Read the model definition and answer for the solid it produces. Units are mm, in the model's axes. A direction names the side the tool comes from. Coordinates: 2 decimals unless noted, no trailing zeros. Write each loop counter-clockwise with the first axis right and the second up, starting at its lowest first coordinate (ties: lowest second). Pieces come first, ordered by that corner, then holes.
Item 1: Each of these flat-tipped pins is pushed along its axis until it touches: P1, Ø10, axis at x = 77, z = -24, coming from the +Y side; P2, Ø1.5, axis at y = 14, z = -18.5, coming from the -X side; P3, Ø21, axis at x = 97, z = -25, coming from the -Y side. Where does it stop, or does it pass through?
Item 2: Straight lines are drawn through the part: probe 1 along X at (y, z) = (48.5, -25); probe 2 along X at (y, z) = (34.25, -25); probe 3 along X at (y, z) = (3, -25). For each, find the intervals that lie inside material, in ascending order.
Item 3: Section C-C (z = -25) is taken. Give the vertices of the cut face in (x, y).
Item 4: Section D-D (x = 28.25) is taken. Give the vertices of the cut face in (y, z).
Item 5: Section A-A (x = 97) is taken. Give the vertices of the cut face in (y, z), then the cut area to 3 significant figures.
Item 6: A tool of negligible diameter and unlimited length cuts with its end or side. For faces 5 (the face through (112.864, 46.084, -27.083)), 6 (the face through (104.3, 12, -28.8)), 7 (the face through (152, 26, -25)), from which of +Z, -Z, +X, -X, +Y, -Y can it reach the whole face along a straight path? Write none if from no direction.
Item 7: Determine the mould class of faces 1 (the face through (92, 26, -50)), 2 (the face through (42, 32, -25)), 3 (the face through (92, 26, 0)), 4 (the face through (112.864, 5.916, -27.083)) for opening direction Z: released by +Z, released by -Z, zero draft, split by the parting line, or undercut.
Item 8: Section B-B (y = 28.5) is taken. Give the vertices of the cut face in (x, z).
from build123d import *

# Parameters (mm, degrees)
SKETCH1_W                = 152
SKETCH1_H                = 52
BOSS_EXTRUDE1_DEPTH      = 50
SKETCH2_W                = 42
SKETCH2_H                = 40
CUT_EXTRUDE1_DEPTH       = 169.249814264
SKETCH3_R                = 16
CUT_EXTRUDE2_DEPTH       = 12
SKETCH4_R                = 8
CUT_EXTRUDE3_DEPTH       = 165.93635136
BOSS_EXTRUDE2_DEPTH      = 10
BOSS_EXTRUDE2_DEPTH_BACK = 40
SKETCH6_R                = 2.5


with BuildPart() as part:
    # Sketch1 → Boss-Extrude1 (new body)
    with BuildSketch(Plane.XY):
        with Locations((76, 26)):
            Rectangle(SKETCH1_W, SKETCH1_H)
    extrude(amount=-BOSS_EXTRUDE1_DEPTH)

    # Sketch2 → Cut-Extrude1 (cut, through all)
    with BuildSketch(Plane.XY):
        with Locations((21, 32)):
            Rectangle(SKETCH2_W, SKETCH2_H)
    extrude(amount=-CUT_EXTRUDE1_DEPTH, mode=Mode.SUBTRACT)

    # Sketch3 → Cut-Extrude2 (cut)
    with BuildSketch(Plane(origin=(0, 52, 0), x_dir=(1, 0, 0), z_dir=(0, 1, 0))):
        with Locations(Location((97, 25, 0), (0, 0, 270))):
            Circle(SKETCH3_R)
    cut_extrude2 = extrude(amount=-CUT_EXTRUDE2_DEPTH, mode=Mode.SUBTRACT)

    # Mirror1: Cut-Extrude2 across plane
    add(cut_extrude2.mirror(Plane.ZX.offset(26)), mode=Mode.SUBTRACT)

    # Sketch4 → Cut-Extrude3 (cut, through all)
    with BuildSketch(Plane(origin=(0, 40, 0), x_dir=(1, 0, 0), z_dir=(0, 1, 0))):
        with Locations(Location((97, 25, 0), (0, 0, 270))):
            Circle(SKETCH4_R)
    extrude(amount=-CUT_EXTRUDE3_DEPTH, mode=Mode.SUBTRACT)

    # Sketch6 → Boss-Extrude2 (add, two sides: drawn at the far end of the back side and taken through both)
    with BuildSketch(Plane(origin=(0, 52, 0), x_dir=(1, 0, 0), z_dir=(0, 1, 0)).offset(-BOSS_EXTRUDE2_DEPTH_BACK)):
        with Locations(Location((28.25, 25, 0), (0, 0, 90))):
            Circle(SKETCH6_R)
    extrude(amount=BOSS_EXTRUDE2_DEPTH + BOSS_EXTRUDE2_DEPTH_BACK)


solid = part.part
Established:
1. P1: stops at y = 52
1. P2: stops at x = 42
1. P3: stops at y = 12
2. probe 1: x = 25.75 to 30.75, 42 to 81, 113 to 152
2. probe 2: x = 25.75 to 30.75, 42 to 89, 105 to 152
2. probe 3: x = 0 to 81, 113 to 152
3. outline: (0, 0) - (81, 0) - (81, 12) - (89, 12) - (89, 40) - (81, 40) - (81, 52) - (42, 52) - (42, 12) - (30.75, 12) - (30.75, 62) - (25.75, 62) - (25.75, 12) - (0, 12) - close; (105, 12) - (113, 12) - (113, 0) - (152, 0) - (152, 52) - (113, 52) - (113, 40) - (105, 40) - close
4. outline: (0, -50) - (12, -50) - (12, -27.5) - (62, -27.5) - (62, -22.5) - (12, -22.5) - (12, 0) - (0, 0) - close
5. outline: (0, -50) - (52, -50) - (52, -41) - (40, -41) - (40, -33) - (12, -33) - (12, -41) - (0, -41) - close; (0, -9) - (12, -9) - (12, -17) - (40, -17) - (40, -9) - (52, -9) - (52, 0) - (0, 0) - close
5. area: 1,380 mm2
6. face 5: +Y
6. face 6: -Y
6. face 7: +Z, -Z, +X, +Y, -Y
7. face 1: released by -Z
7. face 2: zero draft
7. face 3: released by +Z
7. face 4: undercut
8. outline: circle Ø5 at (28.25, -25); (42, -50) - (152, -50) - (152, 0) - (42, 0) - close; hole circle Ø16 at (97, -25)
